Print and shaded views of the part. All mm, measured from the part's lowest x, y and z. A direction names the side the tool comes from. Coordinates: 2 decimals unless noted, no trailing zeros. Loops run counter-clockwise (first coordinate to the right, second up) from the corner with the lowest first, then second, coordinate; pieces in that order, holes last. Notation, with made-up numbers: (-28.5, 49) -> (-2.5, 49) arc R26 ccw to (-2.5, 69) -> close; hole circle Ø1 at (-20.5, 79.5). An arc over 180 degrees is marked (long way). One line per item, written item: value. Start each with the question number.
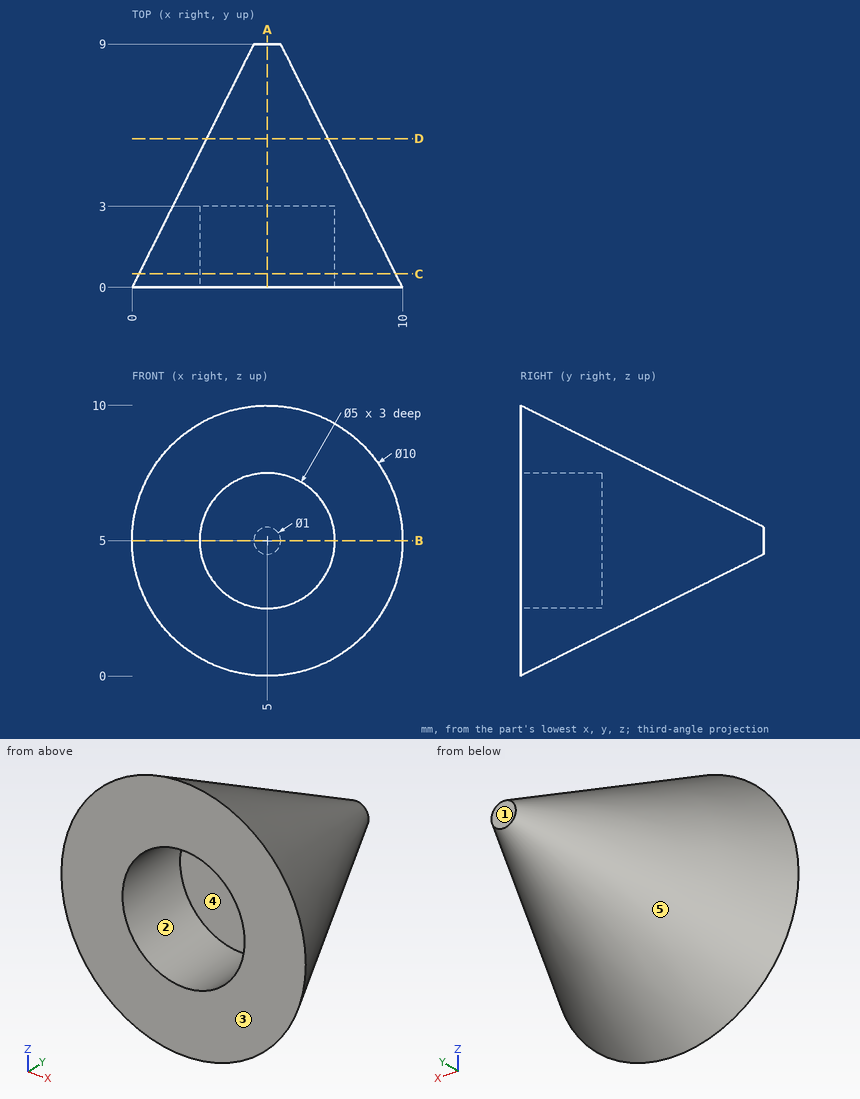
1) Slice it at D-D (y = 5.5). Give the cut face in (x, z), then the cut area to 3 significant figures.
2) Pull direction Z, two halves, no side cores. Call the marked faces 3, 4 and 5: +Z half, -Z half, draft (parallel to the pull), parting line (faces both ways), or undercut.
3) Probe line 1 (Y direction, x = 6, z = 4.25); line 2 (Z direction, x = 5, y = 1.5); line 3 (Z direction, x = 4, y = 2.75). List the from-to ranges inside material, lowest first. Write a range as from..to.
4) Tool access for the marked faces 1 and 2: list every direction of +Z, -Z, +X, -X, +Y, -Y with a clear straight run to the whole face (end or side of a thin tool).
5) Slice it at B-B (z = 5). Give the cut face in (x, y).
6) Slice it at C-C (y = 0.5). Give the cut face in (x, z).
7) Pin check, flat tips, straight feed: pin 1 Ø3 at (x, z) = (8, 7) entering from +Y; pin 2 Ø2.5 at (x, z) = (6, 5.5) entering from -Y; pin 3 Ø5 at (y, z) = (6.5, 5) entering from +X. Stop position of each tip, or through.
8) Slice it at A-A (x = 5). Give the cut face in (y, z).
Check sheet entries:
1. outline: circle Ø4.5 at (5, 5)
1. area: 15.9 mm^2
2. face 3: draft
2. face 4: undercut
2. face 5: parting line
3. line 1: y = 3..7.5
3. line 2: z = 0.75..2.5, 7.5..9.25
3. line 3: z = 1.52..2.71, 7.29..8.48
4. face 1: +Z, -Z, +X, -X, +Y
4. face 2: -Y
5. outline: (0, 0) -> (2.5, 0) -> (2.5, 3) -> (7.5, 3) -> (7.5, 0) -> (10, 0) -> (5.5, 9) -> (4.5, 9) -> close
6. outline: circle Ø9.5 at (5, 5); hole circle Ø5 at (5, 5)
7. pin 1: stops at y = 5.79
7. pin 2: stops at y = 3
7. pin 3: stops at x = 8
8. outline: (0, 0) -> (9, 4.5) -> (9, 5.5) -> (0, 10) -> (0, 7.5) -> (3, 7.5) -> (3, 2.5) -> (0, 2.5) -> close
